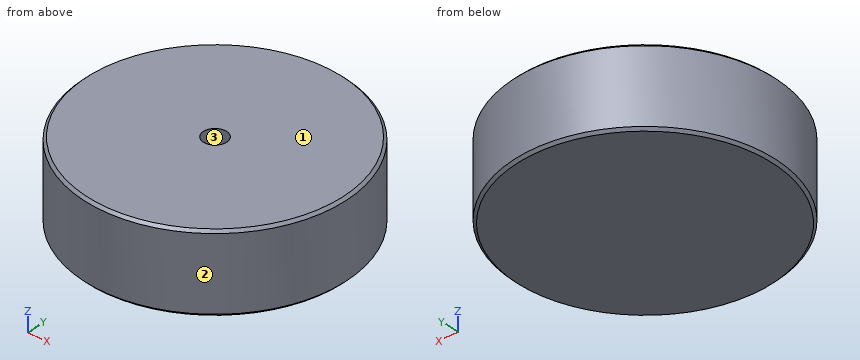
```python
from build123d import *

# Parameters (mm, degrees)
SKETCH1_R                 = 12.7
BOSS_EXTRUDE1_DEPTH       = 7.62
F_4_40_TAPPED_HOLE1_D     = 2.2606
F_4_40_TAPPED_HOLE1_DEPTH = 5.670847242
F_4_40_TAPPED_HOLE1_TIP   = 0.679152758
CHAMFER1_SIZE             = 0.254


with BuildPart() as part:
    # Sketch1 → Boss-Extrude1 (new body)
    with BuildSketch(Plane.XY):
        Circle(SKETCH1_R)
    extrude(amount=BOSS_EXTRUDE1_DEPTH)

    # #4-40 Tapped Hole1
    with Locations(Plane.XY.offset(7.62)):
        with Locations((0, 0)):
            Hole(F_4_40_TAPPED_HOLE1_D / 2, depth=F_4_40_TAPPED_HOLE1_DEPTH)
            with Locations((0, 0, -(F_4_40_TAPPED_HOLE1_DEPTH + F_4_40_TAPPED_HOLE1_TIP / 2))):  # 118° drill point
                Cone(0, F_4_40_TAPPED_HOLE1_D / 2, F_4_40_TAPPED_HOLE1_TIP, mode=Mode.SUBTRACT)

    # Chamfer1
    chamfer1_edges = [part.edges().sort_by_distance(p)[0] for p in [
        (-12.7, 0, 0),
        (-12.7, 0, 7.62),
    ]]
    chamfer(chamfer1_edges, length=CHAMFER1_SIZE)


solid = part.part
```
Build history of the part. All positions in model axes, mm. Face numbers are marked on the shaded views. Round coordinates to 2 decimals unless told otherwise and drop trailing zeros. Loops run counter-clockwise (first coordinate to the right, second up) from the corner with the lowest first, then second, coordinate; pieces in that order, holes last.
Item 1: Drill centre lines: line 1 along Y through (x, z) = (0, 3.95); line 2 along X through (y, z) = (2.5, 4.25); line 3 along Y through (x, z) = (0.75, 6.75). Where is each one in solid material? Low to high.
Item 2: Two-plate mould, pull along Y, no slides. Class the marked faces 1, 2 and 3: released by +Y, released by -Y, zero draft, split by the parting line, or undercut.
Item 3: Saw through at A-A (z = 4.5). List the corners of the cut face in (x, y).
Item 4: Pin check, flat tips, straight feed: P1, Ø1.5, axis at y = -1, z = 5, coming from the -X side; P2, Ø1, axis at x = 3, z = 6, coming from the +Y side; P3, Ø4, axis at x = 3, z = 1, coming from the -Y side. Stop position of each tip, or through.
Worked answers:
1. line 1: y = -12.7 to -1.13, 1.13 to 12.7
1. line 2: x = -12.45 to 12.45
1. line 3: y = -12.68 to -0.85, 0.85 to 12.68
2. face 1: zero draft
2. face 2: split by the parting line
2. face 3: undercut
3. outline: circle Ø25.4 at (0, 0); hole circle Ø2.26 at (0, 0)
4. P1: stops at x = -12.7
4. P2: stops at y = 12.45
4. P3: stops at y = -12.66
